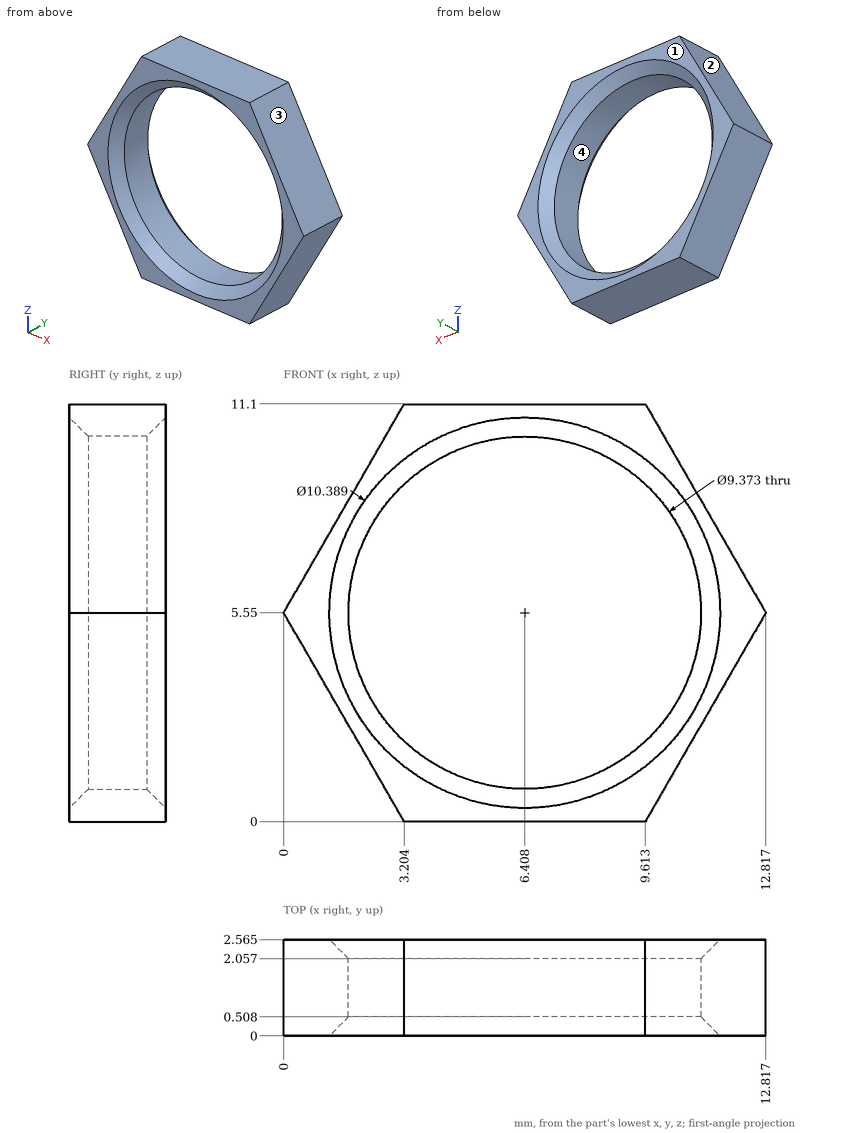
Here's the drawing with two shaded views (mm, measured from the low corner). I have some questions. Give positions to 0.01 mm unless a question says otherwise; leave off trailing zeros. One line per item, written item: value. Start each with the question number.
Item 1: If we mould it in two halves opening along X, with no side actions, what happens to the marked faces 1, 2, 3 and 4? For each: +X half, -X half, draft (parallel to the pull), parting line (faces both ways), or undercut.
Item 2: Please list where these lines run through material, in increasing order: line 1 (Z direction, x = 6.5, y = 1.85) (1 decimal); line 2 (Z direction, x = 8, y = 1.3); line 3 (X direction, y = 1.8, z = 3.5) (1 decimal). Write a range as from..to.
Item 3: I'm going to push flat-ended pins straight in: pin 1 (3 mm diameter, centred on x = 7.5, z = 3.5, fed in from -Y); pin 2 (6 mm diameter, centred on x = 3.5, z = 2.5, fed in from +Y) (1 decimal); pin 3 (1.5 mm diameter, centred on y = 1, z = 2, fed in from +X); pin 4 (1.5 mm diameter, centred on x = 7, z = 9.5, fed in from -Y). Where does each tip first touch, or does it pass through?
Geometry says:
1. face 1: draft
1. face 2: -X half
1. face 3: +X half
1. face 4: undercut
2. line 1: 0..0.9, 10.2..11.1
2. line 2: 0..1.14, 9.96..11.1
2. line 3: 1.2..2.2, 10.6..11.6
3. pin 1: through
3. pin 2: y = 2.6
3. pin 3: x = 11.2
3. pin 4: y = 0.45
